Here's how the part is built. I have some questions about the finished solid (model axes, mm). A direction names the side the tool comes from. Round coordinates to 2 decimals unless told otherwise and drop trailing zeros. Order: outer loops, then holes, each group sorted by start corner. A loop starts at its lowest first (then second) coordinate and runs counter-clockwise, first axis right, second up. Notation, with made-up numbers: (76, -31.75) -> (133, -31.75) arc R25 ccw to (133, 2.25) -> close; hole circle Ø7 at (7, -2). An arc over 180 degrees is marked (long way). Use a Markdown table: item, result. Add a question column.
(1) I'm going to push flat-ended pins straight in: P1, Ø0.8, axis at y = 0.5, z = 8, coming from the -X side; P2, Ø0.8, axis at x = -8, y = 1, coming from the -Z side; P3, Ø0.8, axis at y = 0.5, z = 7.5, coming from the +X side. Where does each tip first touch, or does it pass through?
(2) I want a section at A-A, the plane z = 8. Please give me the cut outline in (x, y), then the cut area to 3 significant figures.
(3) I want a section at C-C, the plane y = 0.85. Please give me the cut outline in (x, z).
(4) If I drill on probe 1 along Z at (x, y) = (-9.5, 1); probe 2 along Z at (x, y) = (3.5, 0.8); probe 3 along X at (y, z) = (1.05, 5.25), over which ranges is the centre line in solid material (lowest first)?
(5) Thinking about a two-plate mould opening in X: for faces 1 (the face through (-4.62, 0.74, -4.57)), 2 (the face through (-6.8, 0.7, 6.7)), 3 (the face through (8, 1, 1.55)), 4 (the face through (-0.1, 0.7, 13.5)), which applies, pulls with the +X half, pulls with the -X half, needs draft (parallel to the pull), parting line crosses it, or undercut?
(6) I want a section at B-B, the plane x = 0. Please give me the cut outline in (y, z), then the cut area to 3 significant figures.
(7) On a 3-axis mill with a long thin cutter (end or side, diameter ignored), from which of +Z, -Z, +X, -X, +Y, -Y can I reach the whole of each face in a straight line? I mean faces 5 (the face through (1.52, 1, -8)), 6 (the face through (-3, 1.5, -6)). Say none if no direction works.
from build123d import *

# Parameters (mm, degrees)
BOSS_EXTRUDE1_DEPTH = 1.5


with BuildPart() as part:
    # Sketch10 → Boss-Extrude1 (new body)
    with BuildSketch(Plane(origin=(0, 0, 0), x_dir=(1, 0, 0), z_dir=(0, 1, 0))):
        with BuildLine():
            ThreePointArc((-9.5, 4), (-13.5, 0), (-9.5, -4))
            Line((-9.5, -4), (-4, -9.5))
            ThreePointArc((-4, -9.5), (0, -13.5), (4, -9.5))
            Line((4, -9.5), (9.5, -4))
            ThreePointArc((9.5, -4), (13.5, 0), (9.5, 4))
            Line((9.5, 4), (4, 9.5))
            ThreePointArc((4, 9.5), (0, 13.5), (-4, 9.5))
            Line((-4, 9.5), (-9.5, 4))
        make_face()
        with BuildLine():
            ThreePointArc((-9.5, -1.55), (-11.05, 0), (-9.5, 1.55))
            Line((-9.5, 1.55), (-6.312487624, 1.55))
            ThreePointArc((-6.312487624, 1.55), (-4.58526578, 4.607096453), (-1.52, 6.319778477))
            Line((-1.52, 6.319778477), (-1.52, 9.5))
            ThreePointArc((-1.52, 9.5), (0, 11.02), (1.52, 9.5))
            Line((1.52, 9.5), (1.52, 6.319778477))
            ThreePointArc((1.52, 6.319778477), (4.58526578, 4.607096453), (6.312487624, 1.55))
            Line((6.312487624, 1.55), (9.5, 1.55))
            ThreePointArc((9.5, 1.55), (11.05, 0), (9.5, -1.55))
            Line((9.5, -1.55), (6.312487624, -1.55))
            ThreePointArc((6.312487624, -1.55), (4.58526578, -4.607096453), (1.52, -6.319778477))
            Line((1.52, -6.319778477), (1.52, -9.5))
            ThreePointArc((1.52, -9.5), (0, -11.02), (-1.52, -9.5))
            Line((-1.52, -9.5), (-1.52, -6.319778477))
            ThreePointArc((-1.52, -6.319778477), (-4.58526578, -4.607096453), (-6.312487624, -1.55))
            Line((-6.312487624, -1.55), (-9.5, -1.55))
        make_face(mode=Mode.SUBTRACT)
    extrude(amount=BOSS_EXTRUDE1_DEPTH)


solid = part.part
Taken from the geometry:
| question | item | result |
|---|---|---|
| 1 | P1 | stops at x = -5.9 |
| 1 | P2 | stops at z = -5.9 |
| 1 | P3 | stops at x = 6.4 |
| 2 | outline | (-5.5, 0) -> (-1.52, 0) -> (-1.52, 1.5) -> (-5.5, 1.5) -> close; (1.52, 0) -> (5.5, 0) -> (5.5, 1.5) -> (1.52, 1.5) -> close |
| 2 | area | 11.9 mm2 |
| 3 | outline | (-9.5, -4) -> (-4, -9.5) arc R4 ccw to (4, -9.5) -> (9.5, -4) arc R4 ccw to (9.5, 4) -> (4, 9.5) arc R4 ccw to (-4, 9.5) -> (-9.5, 4) arc R4 ccw to start; hole (-9.5, -1.55) -> (-6.31, -1.55) arc R6.5 ccw to (-1.52, -6.32) -> (-1.52, -9.5) arc R1.52 ccw to (1.52, -9.5) -> (1.52, -6.32) arc R6.5 ccw to (6.31, -1.55) -> (9.5, -1.55) arc R1.55 ccw to (9.5, 1.55) -> (6.31, 1.55) arc R6.5 ccw to (1.52, 6.32) -> (1.52, 9.5) arc R1.52 ccw to (-1.52, 9.5) -> (-1.52, 6.32) arc R6.5 ccw to (-6.31, 1.55) -> (-9.5, 1.55) arc R1.55 ccw to start |
| 4 | probe 1 | z = -4 to -1.55, 1.55 to 4 |
| 4 | probe 2 | z = -11.44 to -5.48, 5.48 to 11.44 |
| 4 | probe 3 | x = -8.25 to -3.83, 3.83 to 8.25 |
| 5 | face 1 | undercut |
| 5 | face 2 | pulls with the -X half |
| 5 | face 3 | undercut |
| 5 | face 4 | parting line crosses it |
| 6 | outline | (0, -13.5) -> (1.5, -13.5) -> (1.5, -11.02) -> (0, -11.02) -> close; (0, 11.02) -> (1.5, 11.02) -> (1.5, 13.5) -> (0, 13.5) -> close |
| 6 | area | 7.44 mm2 |
| 7 | face 5 | +Y, -Y |
| 7 | face 6 | +Z, -Z, +X, -X, +Y |
